```python
from build123d import *

# Parameters (mm, degrees)
F0_W     = 50
F0_H     = 50
F0_W_2   = 40
F0_H_2   = 40
F1_DEPTH = 20
F2_W     = 50
F2_H     = 50
F3_DEPTH = 25
F4_SIZE  = 24.99999


# Not quite as in the source:
# - a fillet or chamfer is up to 0.001 mm smaller than in the source, because OpenCascade refuses the exact size


with BuildPart() as f1:
    # F0 (on Top) → F1 (new body)
    with BuildSketch(Plane.XY):
        with Locations((25, 25)):
            Rectangle(F0_W, F0_H)
        with Locations((25, 25)):
            Rectangle(F0_W_2, F0_H_2, mode=Mode.SUBTRACT)
    extrude(amount=F1_DEPTH)

    # F2 (on face) → F3 (join)
    with BuildSketch(Plane.XY.offset(20)):
        with Locations((25, 25)):
            Rectangle(F2_W, F2_H)
    extrude(amount=F3_DEPTH)

    # F4 (size 25 in the source; OpenCascade refuses exactly that, so slightly less here)
    f4_edges = [f1.edges().sort_by_distance(p)[0] for p in [
        (0, 25, 45),
        (50, 25, 45),
    ]]
    chamfer(f4_edges, length=F4_SIZE)


solid = f1.part
```
Design review of the part built by this model. Coordinates are the model's own, in mm. A direction names the side the tool comes from. Coordinates: 2 decimals unless noted, no trailing zeros. Write each loop counter-clockwise with the first axis right and the second up, starting at its lowest first coordinate (ties: lowest second). Pieces come first, ordered by that corner, then holes.
1) Machinability: for faces 1 (the flat face through (50, 25, 10)), 2 (the flat face through (25, 45, 10)), which of the approach directions +Z, -Z, +X, -X, +Y, -Y give a long, thin tool a straight path to every point of the face, cutting with its end or side? Answer none if there is none.
2) Add section D-D (z = 21). Write out the cut boundary in (x, y).
3) Add section B-B (z = 9). Write out the cut boundary in (x, y), plus the area to 3 significant figures.
4) To check wall thickness, follow L1, parallel to X at y = 11.5, z = 3.5; L2, parallel to X at y = 3.5, z = 39. State the ranges of each line that lie inside material, in increasing order.
5) Insertion check: pin 1 (1 mm diameter, centred on x = 9.5, y = 11, fed in from +Z); pin 2 (4 mm diameter, centred on y = 39.5, z = 29, fed in from +X); pin 3 (1 mm diameter, centred on x = 29, y = 24, fed in from -Z). Each pin has a flat end and moves straight along its axis. Give the tip position at first contact, or say it passes through.
6) Add section C-C (x = 12). Write out the cut boundary in (y, z), plus the area to 3 significant figures.
Check result:
1. face 1: +Z, -Z, +X, +Y, -Y
1. face 2: -Z
2. outline: (1, 0) - (49, 0) - (49, 50) - (1, 50) - close
3. outline: (0, 0) - (50, 0) - (50, 50) - (0, 50) - close; hole (5, 5) - (45, 5) - (45, 45) - (5, 45) - close
3. area: 900 mm2
4. L1: x = 0 to 5, 45 to 50
4. L2: x = 19 to 31
5. pin 1: stops at z = 30
5. pin 2: stops at x = 43
5. pin 3: stops at z = 20
6. outline: (0, 0) - (5, 0) - (5, 20) - (45, 20) - (45, 0) - (50, 0) - (50, 32) - (0, 32) - close
6. area: 800 mm2
